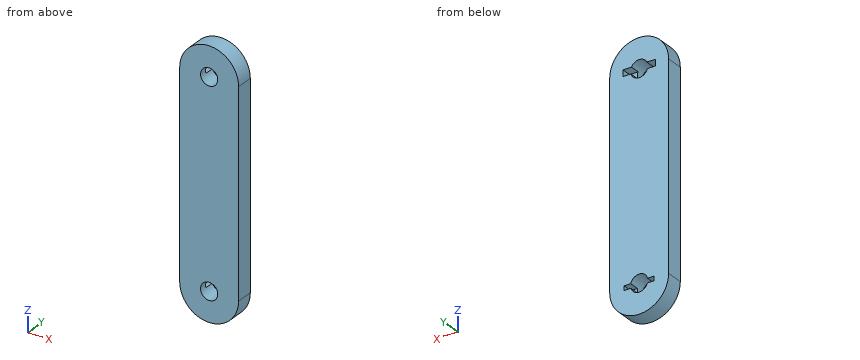
from build123d import *

# Parameters (mm, degrees)
SKETCH1_R           = 3.5
BOSS_EXTRUDE1_DEPTH = 7
SKETCH2_W           = 13.256743243
SKETCH2_H           = 2.580958861
SKETCH2_W_2         = 12.276635078
SKETCH2_H_2         = 1.8
CUT_EXTRUDE1_DEPTH  = 4


with BuildPart() as part:
    # Sketch1 → Boss-Extrude1 (new body)
    with BuildSketch(Plane(origin=(0, 0, 0), x_dir=(1, 0, 0), z_dir=(0, 1, 0))):
        with BuildLine():
            Line((-12, 41.25), (-12, -41.25))
            ThreePointArc((-12, -41.25), (0, -53.25), (12, -41.25))
            Line((12, -41.25), (12, 41.25))
            ThreePointArc((12, 41.25), (0, 53.25), (-12, 41.25))
        make_face()
        with Locations(Location((0, 41.25, 0), (0, 0, 270))):
            Circle(SKETCH1_R, mode=Mode.SUBTRACT)
        with Locations(Location((0, -41.25, 0), (0, 0, 270))):
            Circle(SKETCH1_R, mode=Mode.SUBTRACT)
    extrude(amount=BOSS_EXTRUDE1_DEPTH)

    # Sketch2 → Cut-Extrude1 (cut)
    with BuildSketch(Plane(origin=(0, 7, 0), x_dir=(1, 0, 0), z_dir=(0, 1, 0))):
        with Locations((-0.004439632, -41.523432512)):
            Rectangle(SKETCH2_W, SKETCH2_H)
        with Locations((0, 41.335850456)):
            Rectangle(SKETCH2_W_2, SKETCH2_H_2)
    extrude(amount=-CUT_EXTRUDE1_DEPTH, mode=Mode.SUBTRACT)


solid = part.part
The model under review builds one solid part; all positions refer to its coordinate system, in mm. Coordinates: 2 decimals unless noted, no trailing zeros. Write each loop counter-clockwise with the first axis right and the second up, starting at its lowest first coordinate (ties: lowest second). Pieces come first, ordered by that corner, then holes. Notation, with made-up numbers: (-33.5, 83.25) -> (14.5, 83.25) arc R16 ccw to (14.5, 87.25) -> close; hole circle Ø1 at (79.25, 33). An arc over 180 degrees is marked (long way). Answer in a Markdown table with one row per item.
1. We need section A-A, the plane x = 0. State the section outline as (y, z) points, and give its area (4 significant figures).
Answers below:
| item | result |
|---|---|
| outline | (0, -53.25) -> (7, -53.25) -> (7, -44.75) -> (0, -44.75) -> close; (0, -37.75) -> (7, -37.75) -> (7, 37.75) -> (0, 37.75) -> close; (0, 44.75) -> (7, 44.75) -> (7, 53.25) -> (0, 53.25) -> close |
| area | 647.5 mm^2 |
2. We need section C-C, the plane x = 8.5. State the section outline as (y, z) points.
Answers below:
| item | result |
|---|---|
| outline | (0, -49.72) -> (7, -49.72) -> (7, 49.72) -> (0, 49.72) -> close |
3. Wall thickness on probe 1 along X at (y, z) = (1.5, -41.25); probe 2 along Z at (x, y) = (5.5, 5.25); probe 3 along Z at (x, y) = (2, 1.5): over which ranges is each line inside the solid? List them lowest first. Write a range as [from, to].
Answers below:
| item | result |
|---|---|
| probe 1 | x = [-12, -3.5], [3.5, 12] |
| probe 2 | z = [-51.92, -42.24], [-40.44, 40.23], [42.81, 51.92] |
| probe 3 | z = [-53.08, -44.12], [-38.38, 38.38], [44.12, 53.08] |
4. We need section B-B, the plane y = 2. State the section outline as (x, z) points.
Answers below:
| item | result |
|---|---|
| outline | (-12, -41.25) arc R12 ccw to (12, -41.25) -> (12, 41.25) arc R12 ccw to (-12, 41.25) -> close; hole circle Ø7 at (0, -41.25); hole circle Ø7 at (0, 41.25) |
5. Clearance check with flat-ended pins moving along their axes: pin 1 Ø1.4 at (x, y) = (-4.5, 4) entering from +Z; pin 2 Ø0.9 at (x, z) = (-4.5, -41.5) entering from +Y; pin 3 Ø3 at (x, y) = (6, 4.5) entering from -Z; pin 4 Ø0.9 at (y, z) = (4.5, -41.5) entering from -X. State where each tip first meets the part, or that it passes through.
Answers below:
| item | result |
|---|---|
| pin 1 | stops at z = 52.63 |
| pin 2 | stops at y = 3 |
| pin 3 | stops at z = -52.37 |
| pin 4 | stops at x = -12 |
